```python
from build123d import *

# Parameters (mm, degrees)
F0_W     = 1524
F0_H     = 152.4
F1_DEPTH = 25.4
F2_W     = 25.4
F2_H     = 215.9000692942
F3_DEPTH = 6.35
F4_R     = 3.175
F5_DEPTH = 25.4
F6_START = -127
F6_DEPTH = 25.4


with BuildPart() as f1:
    # F0 (on Top) → F1 (new body)
    with BuildSketch(Plane.XY):
        with Locations((762, 76.2)):
            Rectangle(F0_W, F0_H)
    extrude(amount=F1_DEPTH)

    # F2 (on Top) → F3 (cut)
    with BuildSketch(Plane.XY):
        with Locations((38.1, 77.0159456879)):
            Rectangle(F2_W, F2_H)
        with Locations((520.7, 77.0159456879)):
            Rectangle(F2_W, F2_H)
        with Locations((1003.3, 77.0159456879)):
            Rectangle(F2_W, F2_H)
        with Locations((1485.9, 77.0159456879)):
            Rectangle(F2_W, F2_H)
    extrude(amount=F3_DEPTH, mode=Mode.SUBTRACT)

    # F4 (on Front) → F5 (cut)
    with BuildSketch(Plane.XZ):
        with Locations((101.6, 12.7)):
            Circle(F4_R)
        with Locations((406.4, 12.7)):
            Circle(F4_R)
        with Locations((762, 12.7)):
            Circle(F4_R)
        with Locations((1117.6, 12.7)):
            Circle(F4_R)
        with Locations((1422.4, 12.7)):
            Circle(F4_R)
    extrude(amount=-F5_DEPTH, mode=Mode.SUBTRACT)

    # F4 (on Front) → F6 (cut)
    with BuildSketch(Plane.XZ.offset(F6_START)):
        with Locations((762, 12.7)):
            Circle(F4_R)
        with Locations((1117.6, 12.7)):
            Circle(F4_R)
        with Locations((1422.4, 12.7)):
            Circle(F4_R)
        with Locations((406.4, 12.7)):
            Circle(F4_R)
        with Locations((101.6, 12.7)):
            Circle(F4_R)
    extrude(amount=-F6_DEPTH, mode=Mode.SUBTRACT)


solid = f1.part
```
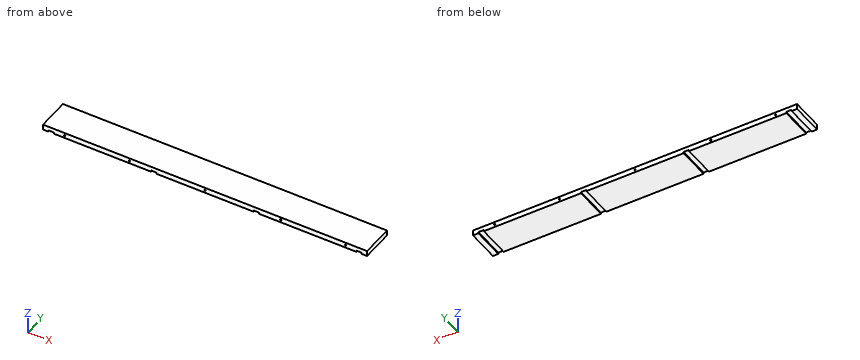
Here's how the part is built. I have some questions about the finished solid (model axes, mm). Give positions to 0.01 mm unless a question says otherwise; leave off trailing zeros. Order: outer loops, then holes, each group sorted by start corner. A loop starts at its lowest first (then second) coordinate and runs counter-clockwise, first axis right, second up. Notation, with made-up numbers: M -15.75,-6.5 L 33.25,-6.5 A27 ccw 33.25,9.5 Z; hole C 42,50 d9. An arc over 180 degrees is marked long. Use a Markdown table: item, result. Add a question column.
1. I need wall thicknesses on probe 1 along X at (y, z) = (83, 5); probe 2 along Z at (x, y) = (1422, 146); probe 3 along X at (y, z) = (146.5, 14). Which ranges of each line are inside material? Lowest first, please. Write a range as from..to.
2. For pin 1 Ø4 at (x, z) = (762, 12.7) entering from +Y; pin 2 Ø5 at (x, z) = (762, 12.7) entering from -Y; pin 3 Ø7.5 at (x, y) = (1481.5, 42) entering from -Z, each with a flat end and sliding along its axis, tell me the tip position at first contact or that it passes through.
3. Suppose I cut it at A-A (y = 104). List the corners of the cut face in (x, z) for me, and give its area (3 significant figures).
Results list:
| question | item | result |
|---|---|---|
| 1 | probe 1 | x = 0..25.4, 50.8..508, 533.4..990.6, 1016..1473.2, 1498.6..1524 |
| 1 | probe 2 | z = 0..9.55, 15.85..25.4 |
| 1 | probe 3 | x = 0..98.7, 104.5..403.5, 409.3..759.1, 764.9..1114.7, 1120.5..1419.5, 1425.3..1524 |
| 2 | pin 1 | stops at y = 127 |
| 2 | pin 2 | stops at y = 25.4 |
| 2 | pin 3 | stops at z = 6.35 |
| 3 | outline | M 0,0 L 25.4,0 L 25.4,6.35 L 50.8,6.35 L 50.8,0 L 508,0 L 508,6.35 L 533.4,6.35 L 533.4,0 L 990.6,0 L 990.6,6.35 L 1016,6.35 L 1016,0 L 1473.2,0 L 1473.2,6.35 L 1498.6,6.35 L 1498.6,0 L 1524,0 L 1524,25.4 L 0,25.4 Z |
| 3 | area | 38,100 mm² |
